For this review, take the finished solid that the model builds, in its own axes (mm). A direction names the side the tool comes from. Round coordinates to 2 decimals unless told otherwise and drop trailing zeros. Write each loop counter-clockwise with the first axis right and the second up, starting at its lowest first coordinate (ties: lowest second). Pieces come first, ordered by that corner, then holes. Notation, with made-up numbers: (4, 10.5) -> (29, 10.5) arc R29 cw to (29, 48.5) -> close; hole circle Ø8 at (36, -0.75). An arc over 180 degrees is marked (long way). Answer as CSV lines item,"result". Start each with the question number.
Item 1: Take a section at D-D on x = 79.5. Give the boundary of the cut face in (y, z).
Item 2: Take a section at C-C on x = 120. Give the boundary of the cut face in (y, z), then the cut area to 3 significant figures.
Item 3: Take a section at B-B on z = 5. Give the boundary of the cut face in (x, y), then the cut area to 3 significant figures.
Item 4: Machinability: for faces 1 (the flat face through (114.439, 39.017, 4.93)), 2 (the cylindrical face through (121.5, 5.07, 5.07)), 3 (the flat face through (63, 6.5, 3)), 4 (the flat face through (131, 6.5, 5)), 5 (the flat face through (89.1, 9.5, 10)), which of the approach directions +Z, -Z, +X, -X, +Y, -Y give a long, thin tool a straight path to every point of the face, cutting with its end or side? Answer none if there is none.
Item 5: For pin 1 Ø2 at (x, z) = (39, 4.5) entering from -Y; pin 2 Ø5 at (y, z) = (49, 3) entering from +X; pin 3 Ø3.5 at (x, z) = (63, 5) entering from +Y, all flat-tipped, find the tip position at first contact; note any pin that passes through.
Item 6: Take a section at A-A on x = 5. Give the boundary of the cut face in (y, z).
Item 7: Mouldability with a two-part tool opening along X and no side actions: class faces 6 (the flat face through (0, 5, 5)), 7 (the flat face through (10, 3, 5)), 8 (the cylindrical face through (6.2, 5.1, 4.1)), 9 (the flat face through (124.777, 39.85, 4.93)) as +X half, -X half, draft (parallel to the pull), parting line (faces both ways), or undercut.
Item 8: Wall thickness on probe 1 along Z at (x, y) = (5, 6.75); probe 2 along Y at (x, z) = (68.5, 2.5); probe 3 along X at (y, z) = (3, 4.25): over which ranges is each line inside the solid? List them lowest first. Write a range as from..to.
```python
from build123d import *

# Parameters (mm, degrees)
PAD_DEPTH    = 10
SKETCH001_R  = 1.5
POCKET_DEPTH = 10.001


with BuildPart() as part:
    # Sketch → Pad (new body)
    with BuildSketch(Plane.XY):
        Polygon((0, 0), (0, 10), (125, 10), (103.577337, 68.858282), (112.974264, 72.278483), (136.915674, 6.5), (125, 6.5), (125, 0), (115, 0), (115, 6.5), (10, 6.5), (10, 0), align=None)
    extrude(amount=PAD_DEPTH)

    # Sketch001 (on Face2 of Pad) → Pocket (cut, through all)
    with BuildSketch(Plane(origin=(0, 10, 0), x_dir=(-1, 0, 0), z_dir=(0, 1, 0))):
        with Locations((-5, 5)):
            Circle(SKETCH001_R)
        with Locations((-120, 5)):
            Circle(SKETCH001_R)
        with Locations((-63, 5)):
            Circle(SKETCH001_R)
    extrude(amount=-POCKET_DEPTH, mode=Mode.SUBTRACT)


solid = part.part
```
Output values:
1,outline,"(6.5, 0) -> (10, 0) -> (10, 10) -> (6.5, 10) -> close"
2,outline,"(0, 0) -> (10, 0) -> (10, 3.5) -> (0, 3.5) -> close; (0, 6.5) -> (10, 6.5) -> (10, 10) -> (0, 10) -> close; (23.74, 0) -> (52.98, 0) -> (52.98, 10) -> (23.74, 10) -> close"
2,area,"362 mm^2"
3,outline,"(0, 0) -> (3.5, 0) -> (3.5, 10) -> (0, 10) -> close; (6.5, 0) -> (10, 0) -> (10, 6.5) -> (61.5, 6.5) -> (61.5, 10) -> (6.5, 10) -> close; (64.5, 6.5) -> (115, 6.5) -> (115, 0) -> (118.5, 0) -> (118.5, 10) -> (64.5, 10) -> close; (103.58, 68.86) -> (125, 10) -> (121.5, 10) -> (121.5, 0) -> (125, 0) -> (125, 6.5) -> (136.92, 6.5) -> (112.97, 72.28) -> close"
3,area,"1,180 mm^2"
4,face 1,"+Z, -Z, -X"
4,face 2,"-Y"
4,face 3,"+Z, -Z, -Y"
4,face 4,"+Z, -Z, +X, -Y"
4,face 5,"+Z, +X, -X, +Y, -Y"
5,pin 1,"stops at y = 6.5"
5,pin 2,"stops at x = 122.36"
5,pin 3,"stops at y = 10"
6,outline,"(0, 0) -> (10, 0) -> (10, 3.5) -> (0, 3.5) -> close; (0, 6.5) -> (10, 6.5) -> (10, 10) -> (0, 10) -> close"
7,face 6,"-X half"
7,face 7,"undercut"
7,face 8,"undercut"
7,face 9,"+X half"
8,probe 1,"z = 0..3.5, 6.5..10"
8,probe 2,"y = 6.5..10"
8,probe 3,"x = 0..3.7, 6.3..10, 115..118.7, 121.3..125"
